Part print with two shaded views. Sizes in mm from the minimum x, y, z corner. Coordinates: 2 decimals unless noted, no trailing zeros. Write each loop counter-clockwise with the first axis right and the second up, starting at its lowest first coordinate (ties: lowest second). Pieces come first, ordered by that corner, then holes. Notation, with made-up numbers: (38, 30.5) - (90, 30.5) arc R10 ccw to (90, 37.5) - close; hole circle Ø8 at (29, -13). An arc over 180 degrees is marked (long way). One line per question, with ' | ' between items. Start each with the question number.
1. Band-saw the part on C-C, the plane x = 4.5. Write the cut outline in (y, z) (1 decimal).
2. Probe line 1 (Z direction, x = 27, y = 1); line 2 (X direction, y = 36.5, z = 7) (1 decimal); line 3 (Z direction, x = 43, y = 8). List the from-to ranges inside material, lowest first.
3. Band-saw the part on D-D, the plane z = 13. Write the cut outline in (x, y).
4. Two-plate mould, pull along Z, no slides. Class the marked faces 1 and 2: +Z half, -Z half, draft (parallel to the pull), parting line (faces both ways), or undercut.
5. Flat gauge pins, fed straight in: P1, Ø8, axis at y = 7.5, z = 18.5, coming from the +X side; P2, Ø1.5, axis at x = 41.5, y = 45, coming from the -Z side; P3, Ø10, axis at x = 21, y = 15.5, coming from the -Z side. Where does each tip first touch, or does it go through?
6. Band-saw the part on A-A, the plane z = 36.5. Write the cut outline in (x, y) (1 decimal).
7. Band-saw the part on B-B, the plane y = 19.5. Write the cut outline in (x, z).
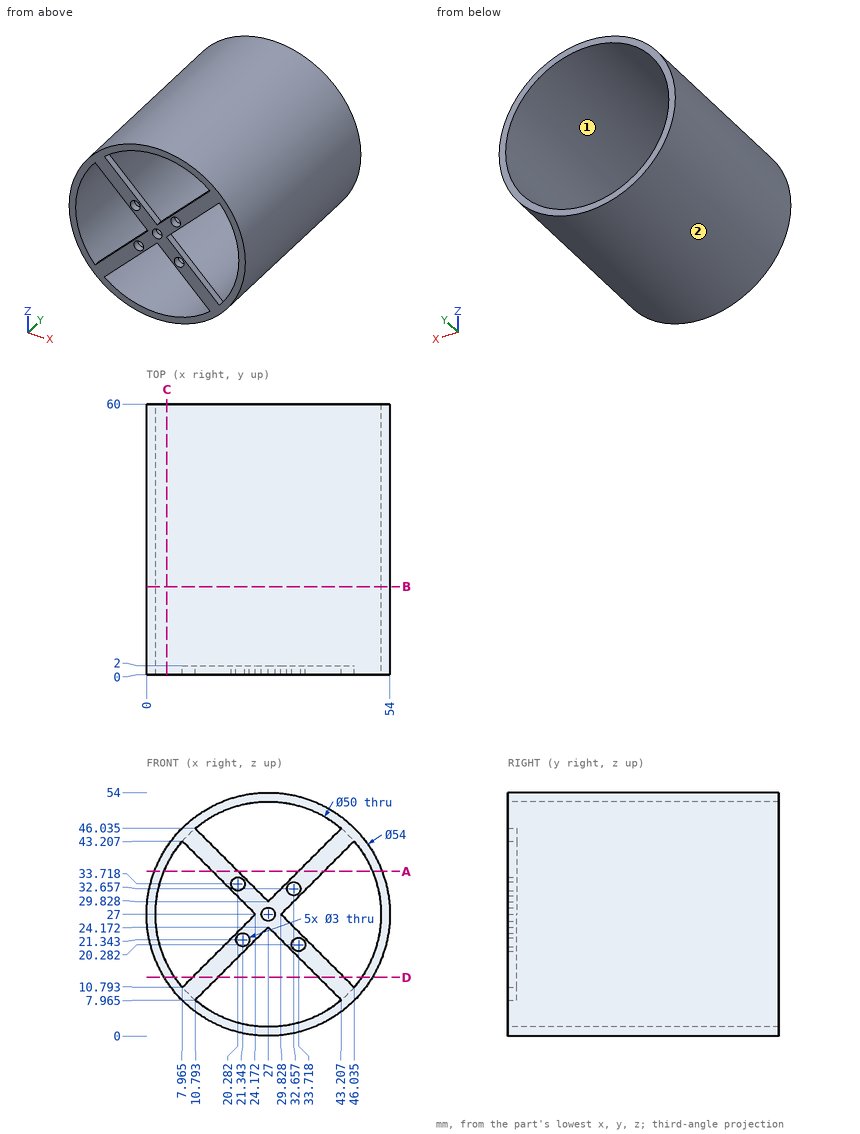
Filled in:
1) outline: (0, 12.1) - (60, 12.1) - (60, 16.1) - (0, 16.1) - close; (0, 37.9) - (60, 37.9) - (60, 41.9) - (0, 41.9) - close
2) line 1: z = 0 to 2, 24.17 to 25.5, 28.5 to 29.83, 52 to 54 | line 2: x = 8.9 to 12, 42 to 45.1 | line 3: z = 5.25 to 7.79, 46.21 to 48.75
3) outline: (3.91, 0) - (6.29, 0) - (6.29, 60) - (3.91, 60) - close; (10.17, 0) - (15.83, 0) - (15.83, 2) - (10.17, 2) - close; (38.17, 0) - (43.83, 0) - (43.83, 2) - (38.17, 2) - close; (47.71, 0) - (50.09, 0) - (50.09, 60) - (47.71, 60) - close
4) face 1: undercut | face 2: parting line
5) P1: stops at x = 53.62 | P2: stops at z = 3.76 | P3: stops at z = 0.02
6) outline: (1.7, 0) - (3.9, 0) - (3.9, 60) - (1.7, 60) - close; (14.7, 0) - (20.3, 0) - (20.3, 2) - (14.7, 2) - close; (33.7, 0) - (39.3, 0) - (39.3, 2) - (33.7, 2) - close; (50.1, 0) - (52.3, 0) - (52.3, 60) - (50.1, 60) - close
7) outline: circle Ø54 at (27, 27); hole circle Ø50 at (27, 27)
